Check sheet for the modelled part. Datum: model origin and axes. Units: mm. Face numbers are marked on the shaded views. A direction names the side the tool comes from. Give positions to 0.01 mm unless a question says otherwise; leave off trailing zeros. Loops run counter-clockwise (first coordinate to the right, second up) from the corner with the lowest first, then second, coordinate; pieces in that order, holes last. Notation, with made-up numbers: (48, -1.75) -> (54, -1.75) arc R13 ccw to (54, 14.25) -> close; hole circle Ø10 at (13, 33). An arc over 180 degrees is marked (long way). Answer as CSV lines item,"result". Start each with the question number.
(1) Material ranges on line 1 (X direction, y = 30, z = 7.5); line 2 (Y direction, x = -64.5, z = 6); line 3 (Y direction, x = -41, z = 2.75), recorded low to high. Write a range as from..to.
(2) Gauge pin test, flat ends, axial feed: pin 1 Ø2 at (y, z) = (11.5, 5) entering from +X; pin 2 Ø4 at (y, z) = (7, 5.5) entering from -X. Record the tip position at first contact, or that the pin passes through.
(3) Section check D-D on x = -49.5. State how many separate pieces and enclosed holes the cut face has, plus the area to 3 significant figures.
(4) Access from +Z, -Z, +X, -X, +Y, -Y to the whole of each face (thin tool, end or side, straight path). Record for the marked faces 4 and 5.
(5) Section check B-B on x = -38. Enter the section's corners in (y, z).
(6) Release check for a two-part mould opening along X. For the marked faces 1, 2 and 3 record: pulls with the +X half, pulls with the -X half, needs draft (parallel to the pull), parting line crosses it, or undercut.
(7) Section check C-C on y = 24. Enter the section's corners in (x, z).
(8) Section check A-A on y = 33.5. Enter the section's corners in (x, z), plus the area to 3 significant figures.
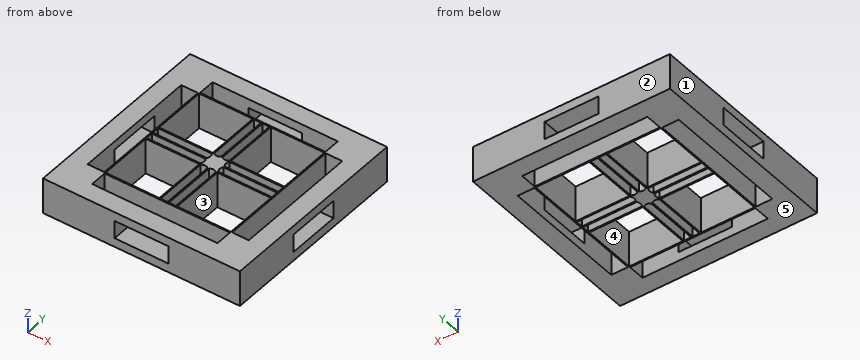
from build123d import *

# Parameters (mm, degrees)
F0_W      = 55
F0_H      = 55
F2_DEPTH  = 10
F1_W      = 35
F1_H      = 4
F1_W_2    = 4
F1_H_2    = 35
F1_W_3    = 15
F1_H_3    = 15
F3_DEPTH  = 25
F4_W      = 1.95
F4_H      = 15
F5_DEPTH  = 25
F6_W      = 1.95
F6_H      = 15
F7_DEPTH  = 25
F8_W      = 15
F8_H      = 1.95
F8_W_2    = 1.95
F8_H_2    = 15
F9_DEPTH  = 25
F10_W     = 35
F10_H     = 4.65
F10_W_2   = 4.65
F10_H_2   = 35
F11_DEPTH = 25
F13_DEPTH = 25
F14_W     = 15.000002
F14_H     = 5
F15_DEPTH = 6
F16_W     = 15
F16_H     = 5
F17_DEPTH = 6
F18_W     = 15
F18_H     = 5
F19_DEPTH = 6
F20_W     = 15
F20_H     = 5
F21_DEPTH = 6


with BuildPart() as f2:
    # F0 (on Top) → F2 (new body)
    with BuildSketch(Plane.XY):
        with Locations((-46.218942, 9.861976)):
            Rectangle(F0_W, F0_H)
    extrude(amount=F2_DEPTH)

    # F1 (on face) → F3 (cut)
    with BuildSketch(Plane.XY):
        with Locations((-46.218942, 30.361976)):
            Rectangle(F1_W, F1_H)
        with Locations((-66.718942, 9.861976)):
            Rectangle(F1_W_2, F1_H_2)
        with Locations((-25.718942, 9.861976)):
            Rectangle(F1_W_2, F1_H_2)
        with Locations((-46.218942, -10.638024)):
            Rectangle(F1_W, F1_H)
        with Locations((-56.218942, 19.861976)):
            Rectangle(F1_W_3, F1_H_3)
        with Locations((-36.218942, 19.861976)):
            Rectangle(F1_W_3, F1_H_3)
        with Locations((-56.218942, -0.138024)):
            Rectangle(F1_W_3, F1_H_3)
        with Locations((-36.218942, -0.138024)):
            Rectangle(F1_W_3, F1_H_3)
    extrude(amount=F3_DEPTH, mode=Mode.SUBTRACT)

    # F4 (on face) → F5 (cut)
    with BuildSketch(Plane.XY.offset(10)):
        with Locations((-47.393942, 19.861976)):
            Rectangle(F4_W, F4_H)
    extrude(amount=-F5_DEPTH, mode=Mode.SUBTRACT)

    # F6 (on face) → F7 (cut)
    with BuildSketch(Plane.XY.offset(10)):
        with Locations((-45.043942, 19.861976)):
            Rectangle(F6_W, F6_H)
    extrude(amount=-F7_DEPTH, mode=Mode.SUBTRACT)

    # F8 (on face) → F9 (cut)
    with BuildSketch(Plane.XY.offset(10)):
        with Locations((-56.218942, 11.036976)):
            Rectangle(F8_W, F8_H)
        with Locations((-56.218942, 8.686976)):
            Rectangle(F8_W, F8_H)
        with Locations((-36.218942, 11.036976)):
            Rectangle(F8_W, F8_H)
        with Locations((-36.218942, 8.686976)):
            Rectangle(F8_W, F8_H)
        with Locations((-47.393942, -0.138024)):
            Rectangle(F8_W_2, F8_H_2)
        with Locations((-45.043942, -0.138024)):
            Rectangle(F8_W_2, F8_H_2)
    extrude(amount=-F9_DEPTH, mode=Mode.SUBTRACT)

    # F10 (on face) → F11 (cut)
    with BuildSketch(Plane.XY.offset(10)):
        with Locations((-46.218942, 30.036976)):
            Rectangle(F10_W, F10_H)
        with Locations((-26.043942, 9.861976)):
            Rectangle(F10_W_2, F10_H_2)
        with Locations((-46.218942, -10.313024)):
            Rectangle(F10_W, F10_H)
        with Locations((-66.393942, 9.861976)):
            Rectangle(F10_W_2, F10_H_2)
    extrude(amount=-F11_DEPTH, mode=Mode.SUBTRACT)

    # F12 (on face) → F13 (cut)
    with BuildSketch(Plane.XY.offset(10)):
        with BuildLine():
            Line((-46.418942, 12.361976), (-48.368942, 12.361976))
            ThreePointArc((-48.368942, 12.361976), (-47.393942, 12.001878), (-46.418942, 12.361976))
        make_face()
        with BuildLine():
            Line((-44.068942, 12.361976), (-46.018942, 12.361976))
            ThreePointArc((-46.018942, 12.361976), (-45.043942, 12.001878), (-44.068942, 12.361976))
        make_face()
        with BuildLine():
            Line((-43.718942, 10.061976), (-43.718942, 12.011976))
            ThreePointArc((-43.718942, 12.011976), (-44.079041, 11.036976), (-43.718942, 10.061976))
        make_face()
        with BuildLine():
            Line((-43.718942, 7.711976), (-43.718942, 9.661976))
            ThreePointArc((-43.718942, 9.661976), (-44.079041, 8.686976), (-43.718942, 7.711976))
        make_face()
        with BuildLine():
            Line((-46.018942, 7.361976), (-44.068942, 7.361976))
            ThreePointArc((-44.068942, 7.361976), (-45.043942, 7.722075), (-46.018942, 7.361976))
        make_face()
        with BuildLine():
            Line((-48.368942, 7.361976), (-46.418942, 7.361976))
            ThreePointArc((-46.418942, 7.361976), (-47.393942, 7.722075), (-48.368942, 7.361976))
        make_face()
        with BuildLine():
            Line((-48.718942, 9.661976), (-48.718942, 7.711976))
            ThreePointArc((-48.718942, 7.711976), (-48.358843, 8.686976), (-48.718942, 9.661976))
        make_face()
        with BuildLine():
            Line((-48.718942, 12.011976), (-48.718942, 10.061976))
            ThreePointArc((-48.718942, 10.061976), (-48.358843, 11.036976), (-48.718942, 12.011976))
        make_face()
    extrude(amount=-F13_DEPTH, mode=Mode.SUBTRACT)

    # F14 (on face) → F15 (cut)
    with BuildSketch(Plane.XZ.offset(17.638024)):
        with Locations((-46.218943, 5)):
            Rectangle(F14_W, F14_H)
    extrude(amount=-F15_DEPTH, mode=Mode.SUBTRACT)

    # F16 (on face) → F17 (cut)
    with BuildSketch(Plane.YZ.offset(-18.718942)):
        with Locations((9.861976, 5)):
            Rectangle(F16_W, F16_H)
    extrude(amount=-F17_DEPTH, mode=Mode.SUBTRACT)

    # F18 (on face) → F19 (cut)
    with BuildSketch(Plane(origin=(0, 37.361976, 0), x_dir=(-1, 0, 0), z_dir=(0, 1, 0))):
        with Locations((46.218942, 5)):
            Rectangle(F18_W, F18_H)
    extrude(amount=-F19_DEPTH, mode=Mode.SUBTRACT)

    # F20 (on face) → F21 (cut)
    with BuildSketch(Plane(origin=(-73.718942, 0, 0), x_dir=(0, -1, 0), z_dir=(-1, 0, 0))):
        with Locations((-9.861976, 5.117217)):
            Rectangle(F20_W, F20_H)
    extrude(amount=-F21_DEPTH, mode=Mode.SUBTRACT)


solid = f2.part
Working result:
1,line 1,"x = -73.72..-63.72, -28.72..-18.72"
1,line 2,"y = -17.64..-7.64, 27.36..37.36"
1,line 3,"y = -7.99..-7.64, 7.36..7.71, 9.66..10.06, 12.01..12.36, 27.36..27.71"
2,pin 1,"stops at x = -28.37"
2,pin 2,"stops at x = -64.07"
3,separate pieces,"9"
3,enclosed holes,"0"
3,area,"68.0 mm^2"
4,face 4,"+Z, -Z"
4,face 5,"-Z, +X, -X, +Y, -Y"
5,outline,"(-17.64, 0) -> (-12.64, 0) -> (-12.64, 10) -> (-17.64, 10) -> close; (-7.99, 0) -> (-7.64, 0) -> (-7.64, 10) -> (-7.99, 10) -> close; (7.36, 0) -> (7.71, 0) -> (7.71, 10) -> (7.36, 10) -> close; (9.66, 0) -> (10.06, 0) -> (10.06, 10) -> (9.66, 10) -> close; (12.01, 0) -> (12.36, 0) -> (12.36, 10) -> (12.01, 10) -> close; (27.36, 0) -> (27.71, 0) -> (27.71, 10) -> (27.36, 10) -> close; (32.36, 0) -> (37.36, 0) -> (37.36, 10) -> (32.36, 10) -> close"
6,face 1,"pulls with the -X half"
6,face 2,"needs draft"
6,face 3,"undercut"
7,outline,"(-73.72, 0) -> (-68.72, 0) -> (-68.72, 10) -> (-73.72, 10) -> close; (-64.07, 0) -> (-63.72, 0) -> (-63.72, 10) -> (-64.07, 10) -> close; (-48.72, 0) -> (-48.37, 0) -> (-48.37, 10) -> (-48.72, 10) -> close; (-46.42, 0) -> (-46.02, 0) -> (-46.02, 10) -> (-46.42, 10) -> close; (-44.07, 0) -> (-43.72, 0) -> (-43.72, 10) -> (-44.07, 10) -> close; (-28.72, 0) -> (-28.37, 0) -> (-28.37, 10) -> (-28.72, 10) -> close; (-23.72, 0) -> (-18.72, 0) -> (-18.72, 10) -> (-23.72, 10) -> close"
8,outline,"(-73.72, 0) -> (-18.72, 0) -> (-18.72, 10) -> (-73.72, 10) -> close; hole (-53.72, 2.5) -> (-38.72, 2.5) -> (-38.72, 7.5) -> (-53.72, 7.5) -> close"
8,area,"475 mm^2"
